Read the model definition and answer for the solid it produces. Units are mm, in the model's axes. Coordinates: 2 decimals unless noted, no trailing zeros. Write each loop counter-clockwise with the first axis right and the second up, starting at its lowest first coordinate (ties: lowest second). Pieces come first, ordered by that corner, then holes. Notation, with made-up numbers: (-5.75, 80) -> (9.25, 80) arc R36 ccw to (9.25, 119) -> close; hole circle Ø5 at (74.25, 45.5). An arc over 180 degrees is marked (long way). Answer as a JSON object with one key per item and string values. Group by question number.
(1) For a pull along Y with two mould halves and no side action, classify faces 1 (the face through (-5.761, 132.375, 14.79)), 2 (the face through (60, -119, 0)) as +Y half, -Y half, draft (parallel to the pull), parting line (faces both ways), or undercut.
(2) Flat-ended cylindrical pins translate along their axes: P1, Ø10, axis at x = -80, z = 22, coming from the -Y side; P2, Ø8, axis at y = 80.5, z = 13.5, coming from the +X side; P3, Ø5, axis at x = -9.5, z = 17, coming from the -Y side. Find the tip coordinate at first contact, or state that the pin passes through.
(3) Find section B-B (x = 101). Give the vertices of the cut face in (y, z), then the cut area to 3 significant figures.
(4) Find section A-A (y = 0). Give the vertices of the cut face in (x, z).
(5) Find section C-C (z = 8). Give the vertices of the cut face in (x, y), then the cut area to 3 significant figures.
(6) Straight lines are drawn through the part: L1, parallel to X at y = 0, z = 14.25; L2, parallel to Y at x = -40, z = 16.75; L3, parallel to Y at x = 44.5, z = 10. For each, find the intervals that lie inside material, in ascending order.
Autodesk Inventor part; units mm, degrees
ref_plane "YZ Plane" through (0, 0, 0) normal (1, 0, 0) x (0, 1, 0)
ref_plane "XZ Plane" through (0, 0, 0) normal (0, 1, 0) x (-1, 0, 0)
ref_plane "XY Plane" through (0, 0, 0) normal (0, 0, 1) x (1, 0, 0)
sketch "스케치1" plane through (0, 0, 0) normal (0, 0, 1) x (1, 0, 0)
  arc A0 (4.6242, -132.4193) -> (-4.6242, -132.4193) centre (0, 0) ccw
  arc A1 (4.7289, -135.4175) -> (-4.7289, -135.4175) centre (0, 0) ccw
  line L0 (0, 0) -> (-4.7289, -135.4175)
  line L1 (0, 0) -> (135.5, 0) construction
  line L2 (0, 0) -> (4.7289, -135.4175)
  line L3 (0, 0) -> (135.5, 0) construction
  line L4 (-4.7289, -135.4175) -> (-5.0779, -145.4114)
  line L5 (-5.0779, -145.4114) -> (-7.0767, -145.3416)
  line L6 (-7.0767, -145.3416) -> (-6.7271, -135.3329)
  line L7 (4.7289, -135.4175) -> (5.0779, -145.4114)
  line L8 (4.7289, -135.4175) -> (14.7289, -135.4175) construction
  line L9 (5.0779, -145.4114) -> (7.0767, -145.3416)
  line L10 (7.0767, -145.3416) -> (6.7271, -135.3329)
  dimension "d0" = 265
  dimension "d1" = 3
  dimension "d2" = 92
  dimension "d3" = 88
  dimension "d4" = 10
  dimension "d5" = 2
  dimension "d6" = 90
  dimension "d7" = 90
  dimension "d8" = 10
  dimension "d9" = 88
  dimension "d10" = 2
  dimension "d11" = 90
  dimension "d12" = 90
extrude "돌출1" add sketch "스케치1" along normal blind 30 contours A0 L0 A1 L2 | A1 L10 L9 L7 | L4 L5 L6 A1
sketch "스케치2" plane through (6.7271, -135.3329, 30) normal (0.9994, 0.0349, 0) x (0, 0, -1)
  line L0 (30, -10.0148) -> (0, -10.0148)
  line L1 (15, -10.0148) -> (15, -5.0148)
  circle A0 centre (15, -5.0148) radius 2.6
  point P0 (30, 135.4852)
  dimension "d15" = 5
  dimension "d16" = 5.2
extrude "돌출2" cut sketch "스케치2" against normal up to surface (2 mm away)
sketch "스케치3" plane through (-7.0767, -145.3416, 0) normal (-0.9994, 0.0349, 0) x (0, 0, 1)
  line L0 (0, 0) -> (30, 0)
  line L1 (15, 0) -> (15, 5)
  line L2 (15, 0) -> (20, 0) construction
  circle A0 centre (15, 5) radius 2.6
  point P0 (0, 145.5)
  dimension "d19" = 5
  dimension "d20" = 90
  dimension "d21" = 5.2
extrude "돌출3" cut sketch "스케치3" against normal up to surface (2 mm away)
properties part number "camera_robotarm"
Results below:
{
 "1": {"face 1": "undercut", "face 2": "draft"},
 "2": {"P1": "stops at y = -112.85", "P2": "stops at x = 111.84", "P3": "stops at y = -145.34"},
 "3": {"outline": "(-90.33, 0) -> (-85.76, 0) -> (-85.76, 30) -> (-90.33, 30) -> close; (85.76, 0) -> (90.33, 0) -> (90.33, 30) -> (85.76, 30) -> close", "area": "274 mm2"},
 "4": {"outline": "(-135.5, 0) -> (-132.5, 0) -> (-132.5, 30) -> (-135.5, 30) -> close; (132.5, 0) -> (135.5, 0) -> (135.5, 30) -> (132.5, 30) -> close"},
 "5": {"outline": "(-7.08, -145.34) -> (-5.08, -145.41) -> (-4.73, -135.42) -> (-4.62, -132.42) arc R132.5 cw (long way) to (4.62, -132.42) -> (4.73, -135.42) -> (5.08, -145.41) -> (7.08, -145.34) -> (6.73, -135.33) arc R135.5 ccw (long way) to (-6.73, -135.33) -> close", "area": "2,540 mm2"},
 "6": {"L1": "x = -135.5 to -132.5, 132.5 to 135.5", "L2": "y = -129.46 to -126.32, 126.32 to 129.46", "L3": "y = -127.98 to -124.8, 124.8 to 127.98"}
}
